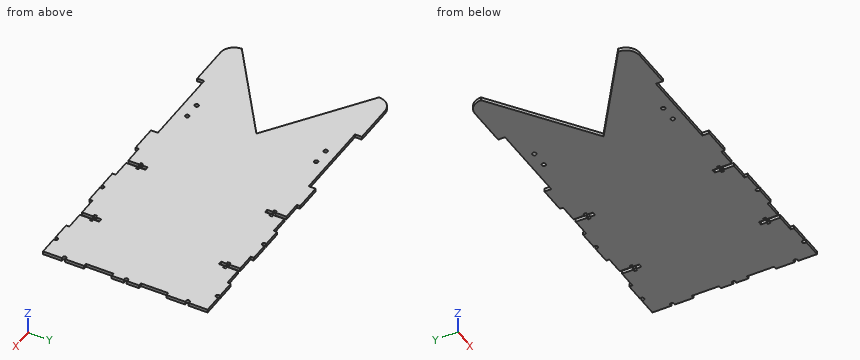
```python
from build123d import *

# Parameters (mm, degrees)
F0_R     = 1.8161
F1_DEPTH = 2.9718


with BuildPart() as f1:
    # F0 (on Top) → F1 (new body)
    with BuildSketch(Plane.XY):
        with BuildLine():
            Line((134.594341, -76.2), (152.4, -76.2))
            Line((152.4, -76.2), (152.4, -58.394341))
            ThreePointArc((152.4, -58.394341), (149.352, -57.15), (152.4, -55.905659))
            Line((152.4, -55.905659), (152.4, -38.1))
            Line((152.4, -38.1), (149.4282, -38.1))
            Line((149.4282, -38.1), (149.4282, -12.7))
            Line((149.4282, -12.7), (152.4, -12.7))
            Line((152.4, -12.7), (152.4, -1.244341))
            ThreePointArc((152.4, -1.244341), (149.352, 0), (152.4, 1.244341))
            Line((152.4, 1.244341), (152.4, 12.7))
            Line((152.4, 12.7), (149.4282, 12.7))
            Line((149.4282, 12.7), (149.4282, 38.1))
            Line((149.4282, 38.1), (152.4, 38.1))
            Line((152.4, 38.1), (152.4, 55.905659))
            ThreePointArc((152.4, 55.905659), (149.352, 57.15), (152.4, 58.394341))
            Line((152.4, 58.394341), (152.4, 76.2))
            Line((152.4, 76.2), (134.594341, 76.2))
            ThreePointArc((134.594341, 76.2), (133.35, 73.152), (132.105659, 76.2))
            Line((132.105659, 76.2), (114.3, 76.2))
            Line((114.3, 76.2), (114.3, 73.2282))
            Line((114.3, 73.2282), (97.0153, 73.2282))
            Line((97.0153, 73.2282), (97.0153, 63.0682))
            Line((97.0153, 63.0682), (99.1362, 63.0682))
            Line((99.1362, 63.0682), (99.1362, 60.4266))
            Line((99.1362, 60.4266), (97.0153, 60.4266))
            Line((97.0153, 60.4266), (97.0153, 55.3974))
            Line((97.0153, 55.3974), (93.4847, 55.3974))
            Line((93.4847, 55.3974), (93.4847, 60.4266))
            Line((93.4847, 60.4266), (91.3638, 60.4266))
            Line((91.3638, 60.4266), (91.3638, 63.0682))
            Line((91.3638, 63.0682), (93.4847, 63.0682))
            Line((93.4847, 63.0682), (93.4847, 73.2282))
            Line((93.4847, 73.2282), (76.2, 73.2282))
            Line((76.2, 73.2282), (76.2, 76.2))
            Line((76.2, 76.2), (58.394341, 76.2))
            ThreePointArc((58.394341, 76.2), (57.15, 73.152), (55.905659, 76.2))
            Line((55.905659, 76.2), (38.1, 76.2))
            Line((38.1, 76.2), (38.1, 73.2282))
            Line((38.1, 73.2282), (20.8153, 73.2282))
            Line((20.8153, 73.2282), (20.8153, 63.0682))
            Line((20.8153, 63.0682), (22.9362, 63.0682))
            Line((22.9362, 63.0682), (22.9362, 60.4266))
            Line((22.9362, 60.4266), (20.8153, 60.4266))
            Line((20.8153, 60.4266), (20.8153, 55.3974))
            Line((20.8153, 55.3974), (17.2847, 55.3974))
            Line((17.2847, 55.3974), (17.2847, 60.4266))
            Line((17.2847, 60.4266), (15.1638, 60.4266))
            Line((15.1638, 60.4266), (15.1638, 63.0682))
            Line((15.1638, 63.0682), (17.2847, 63.0682))
            Line((17.2847, 63.0682), (17.2847, 73.2282))
            Line((17.2847, 73.2282), (0, 73.2282))
            Line((0, 73.2282), (0, 76.2))
            Line((0, 76.2), (-25.4, 76.2))
            Line((-25.4, 76.2), (-25.4, 69.85))
            Line((-25.4, 69.85), (-101.6, 69.85))
            Line((-101.6, 69.85), (-101.6, 76.2))
            Line((-101.6, 76.2), (-139.7, 76.2))
            ThreePointArc((-139.7, 76.2), (-148.680256, 72.480256), (-152.4, 63.5))
            Line((-152.4, 63.5), (-63.5, 0))
            Line((-63.5, 0), (-152.4, -63.5))
            ThreePointArc((-152.4, -63.5), (-148.680256, -72.480256), (-139.7, -76.2))
            Line((-139.7, -76.2), (-101.6, -76.2))
            Line((-101.6, -76.2), (-101.6, -69.85))
            Line((-101.6, -69.85), (-25.4, -69.85))
            Line((-25.4, -69.85), (-25.4, -76.2))
            Line((-25.4, -76.2), (0, -76.2))
            Line((0, -76.2), (0, -73.2282))
            Line((0, -73.2282), (17.2847, -73.2282))
            Line((17.2847, -73.2282), (17.2847, -63.0682))
            Line((17.2847, -63.0682), (15.1638, -63.0682))
            Line((15.1638, -63.0682), (15.1638, -60.4266))
            Line((15.1638, -60.4266), (17.2847, -60.4266))
            Line((17.2847, -60.4266), (17.2847, -55.3974))
            Line((17.2847, -55.3974), (20.8153, -55.3974))
            Line((20.8153, -55.3974), (20.8153, -60.4266))
            Line((20.8153, -60.4266), (22.9362, -60.4266))
            Line((22.9362, -60.4266), (22.9362, -63.0682))
            Line((22.9362, -63.0682), (20.8153, -63.0682))
            Line((20.8153, -63.0682), (20.8153, -73.2282))
            Line((20.8153, -73.2282), (38.1, -73.2282))
            Line((38.1, -73.2282), (38.1, -76.2))
            Line((38.1, -76.2), (55.905659, -76.2))
            ThreePointArc((55.905659, -76.2), (57.15, -73.152), (58.394341, -76.2))
            Line((58.394341, -76.2), (76.2, -76.2))
            Line((76.2, -76.2), (76.2, -73.2282))
            Line((76.2, -73.2282), (93.4847, -73.2282))
            Line((93.4847, -73.2282), (93.4847, -63.0682))
            Line((93.4847, -63.0682), (91.3638, -63.0682))
            Line((91.3638, -63.0682), (91.3638, -60.4266))
            Line((91.3638, -60.4266), (93.4847, -60.4266))
            Line((93.4847, -60.4266), (93.4847, -55.3974))
            Line((93.4847, -55.3974), (97.0153, -55.3974))
            Line((97.0153, -55.3974), (97.0153, -60.4266))
            Line((97.0153, -60.4266), (99.1362, -60.4266))
            Line((99.1362, -60.4266), (99.1362, -63.0682))
            Line((99.1362, -63.0682), (97.0153, -63.0682))
            Line((97.0153, -63.0682), (97.0153, -73.2282))
            Line((97.0153, -73.2282), (114.3, -73.2282))
            Line((114.3, -73.2282), (114.3, -76.2))
            Line((114.3, -76.2), (132.105659, -76.2))
            ThreePointArc((132.105659, -76.2), (133.35, -73.152), (134.594341, -76.2))
        make_face()
        with Locations((-71.3105, -59.69)):
            Circle(F0_R, mode=Mode.SUBTRACT)
        with Locations((-55.6895, -59.69)):
            Circle(F0_R, mode=Mode.SUBTRACT)
        with Locations((-71.3105, 59.69)):
            Circle(F0_R, mode=Mode.SUBTRACT)
        with Locations((-55.6895, 59.69)):
            Circle(F0_R, mode=Mode.SUBTRACT)
    extrude(amount=F1_DEPTH)


solid = f1.part
```
Geometry check sheet. Reference: the model listing, model coordinates, mm. Give positions to 0.01 mm unless a question says otherwise; leave off trailing zeros. Order: outer loops, then holes, each group sorted by start corner. A loop starts at its lowest first (then second) coordinate and runs counter-clockwise, first axis right, second up. Notation, with made-up numbers: (2, -32) - (37, -32) arc R23 ccw to (37, -19) - close; hole circle Ø2 at (-14, 45.5). An arc over 180 degrees is marked (long way). Write item = value, one per line. Start each with the question number.
1) Section check B-B (z = 2.25). Count the separate pieces of the cut face and the enclosed holes in it, then the cut area to 3 significant figures.
2) Section check A-A (x = -88). Enter the section's corners in (y, z), then the cut area to 3 significant figures.
3) Scan lines: L1, parallel to Y at x = 151.13, z = 1.65; L2, parallel to Y at x = -71.5, z = 0.7; L3, parallel to X at y = 68, z = 1.65. Record each from-to range of solid material in increasing order.
4) Section check D-D (x = -128). Enter the section's corners in (y, z), then the cut area to 3 significant figures.
5) Section check C-C (y = -42.5). Enter the section's corners in (x, z), then the cut area to 3 significant figures.
6) Gauge pin test, flat ends, axial feed: pin 1 Ø1.1 at (x, z) = (98, 1.5) entering from -Y; pin 2 Ø1.5 at (y, z) = (-74.5, 1) entering from -X; pin 3 Ø1.7 at (x, z) = (98, 1.5) entering from +Y. Record the tip position at first contact, or that the pin passes through.
Geometry check:
q1.separate_pieces = 1
q1.enclosed_holes = 4
q1.area = 38,800 mm2
q2.outline = (-69.85, 0) - (-17.5, 0) - (-17.5, 2.97) - (-69.85, 2.97) - close; (17.5, 0) - (69.85, 0) - (69.85, 2.97) - (17.5, 2.97) - close
q2.area = 311 mm2
q3.L1 = -76.2 to -58.93, -55.37 to -38.1, -12.7 to -1.78, 1.78 to 12.7, 38.1 to 55.37, 58.93 to 76.2
q3.L2 = -69.85 to -61.5, -57.88 to -5.71, 5.71 to 57.88, 61.5 to 69.85
q3.L3 = -151.58 to 17.28, 20.82 to 93.48, 97.02 to 152.4
q4.outline = (-76.2, 0) - (-46.07, 0) - (-46.07, 2.97) - (-76.2, 2.97) - close; (46.07, 0) - (76.2, 0) - (76.2, 2.97) - (46.07, 2.97) - close
q4.area = 179 mm2
q5.outline = (-123, 0) - (152.4, 0) - (152.4, 2.97) - (-123, 2.97) - close
q5.area = 818 mm2
q6.pin_1 = -73.23
q6.pin_2 = -147.2
q6.pin_3 = 73.23
